from build123d import *

# Parameters (mm, degrees)
SK_BACK_PLATE_W         = 90
SK_BACK_PLATE_H         = 70
SK_BACK_PLATE_R         = 2.25
SK_BACK_PLATE_R_2       = 6
BACK_PLATE_DEPTH        = 8
SK_ROLL_PILOT_RECESS_R  = 22.15
ROLL_PILOT_RECESS_DEPTH = 2.2
SK_MEDIAL_PLATE_R       = 2.75
SK_MEDIAL_PLATE_R_2     = 13
MEDIAL_PLATE_DEPTH      = 8


with BuildPart() as part:
    # SK_Back_Plate → Back_Plate (new body)
    with BuildSketch(Plane(origin=(-76, 0, 0), x_dir=(0, 0, -1), z_dir=(1, 0, 0))):
        with Locations((0, -1)):
            Rectangle(SK_BACK_PLATE_W, SK_BACK_PLATE_H)
        with Locations((25.86862691, 10.715136106)):
            Circle(SK_BACK_PLATE_R, mode=Mode.SUBTRACT)
        with Locations((10.715136106, 25.86862691)):
            Circle(SK_BACK_PLATE_R, mode=Mode.SUBTRACT)
        with Locations((-10.715136106, 25.86862691)):
            Circle(SK_BACK_PLATE_R, mode=Mode.SUBTRACT)
        with Locations((-25.86862691, 10.715136106)):
            Circle(SK_BACK_PLATE_R, mode=Mode.SUBTRACT)
        with Locations((-25.86862691, -10.715136106)):
            Circle(SK_BACK_PLATE_R, mode=Mode.SUBTRACT)
        with Locations((-10.715136106, -25.86862691)):
            Circle(SK_BACK_PLATE_R, mode=Mode.SUBTRACT)
        with Locations((10.715136106, -25.86862691)):
            Circle(SK_BACK_PLATE_R, mode=Mode.SUBTRACT)
        with Locations((25.86862691, -10.715136106)):
            Circle(SK_BACK_PLATE_R, mode=Mode.SUBTRACT)
        Circle(SK_BACK_PLATE_R_2, mode=Mode.SUBTRACT)
    extrude(amount=BACK_PLATE_DEPTH)

    # SK_Roll_Pilot_Recess → Roll_Pilot_Recess (cut)
    with BuildSketch(Plane(origin=(-76, 0, 0), x_dir=(0, 0, -1), z_dir=(1, 0, 0))):
        Circle(SK_ROLL_PILOT_RECESS_R)
    extrude(amount=ROLL_PILOT_RECESS_DEPTH, mode=Mode.SUBTRACT)

    # SK_Medial_Plate → Medial_Plate (add)
    with BuildSketch(Plane(origin=(0, -28, 0), x_dir=(1, 0, 0), z_dir=(0, 1, 0))):
        Polygon((-68, 56), (30, 56), (56, 30), (56, -30), (30, -56), (-68, -56), align=None)
        with Locations(Location((46.193976626, 19.134171618, 0), (0, 0, 270))):
            Circle(SK_MEDIAL_PLATE_R, mode=Mode.SUBTRACT)
        with Locations(Location((19.134171618, 46.193976626, 0), (0, 0, 270))):
            Circle(SK_MEDIAL_PLATE_R, mode=Mode.SUBTRACT)
        with Locations(Location((-19.134171618, 46.193976626, 0), (0, 0, 270))):
            Circle(SK_MEDIAL_PLATE_R, mode=Mode.SUBTRACT)
        with Locations(Location((-46.193976626, 19.134171618, 0), (0, 0, 270))):
            Circle(SK_MEDIAL_PLATE_R, mode=Mode.SUBTRACT)
        with Locations(Location((-46.193976626, -19.134171618, 0), (0, 0, 270))):
            Circle(SK_MEDIAL_PLATE_R, mode=Mode.SUBTRACT)
        with Locations(Location((-19.134171618, -46.193976626, 0), (0, 0, 270))):
            Circle(SK_MEDIAL_PLATE_R, mode=Mode.SUBTRACT)
        with Locations(Location((19.134171618, -46.193976626, 0), (0, 0, 270))):
            Circle(SK_MEDIAL_PLATE_R, mode=Mode.SUBTRACT)
        with Locations(Location((46.193976626, -19.134171618, 0), (0, 0, 270))):
            Circle(SK_MEDIAL_PLATE_R, mode=Mode.SUBTRACT)
        with Locations(Location((0, 0, 0), (0, 0, 270))):
            Circle(SK_MEDIAL_PLATE_R_2, mode=Mode.SUBTRACT)
    extrude(amount=MEDIAL_PLATE_DEPTH)


solid = part.part
Could you check a few things on this model? Use its own coordinates, in mm. A direction names the side the tool comes from. Round coordinates to 2 decimals unless told otherwise and drop trailing zeros. Order: outer loops, then holes, each group sorted by start corner. A loop starts at its lowest first (then second) coordinate and runs counter-clockwise, first axis right, second up.
(1) Imagine slicing it at D-D (z = -33). Write out the boundary of the cut face in (x, y).
Response values:
outline: (-76, -36) - (-68, -36) - (-68, -28) - (53, -28) - (53, -20) - (-68, -20) - (-68, 34) - (-76, 34) - close
(2) Imagine slicing it at A-A (y = 0). Write out the boundary of the cut face in (x, z), plus the area to 3 significant figures.
Response values:
outline: (-76, -45) - (-68, -45) - (-68, -6) - (-73.8, -6) - (-73.8, -22.15) - (-76, -22.15) - close; (-76, 22.15) - (-73.8, 22.15) - (-73.8, 6) - (-68, 6) - (-68, 45) - (-76, 45) - close
area: 553 mm2
(3) Imagine slicing it at B-B (z = 0). Write out the boundary of the cut face in (x, y).
Response values:
outline: (-76, -36) - (-68, -36) - (-68, -28) - (-13, -28) - (-13, -20) - (-68, -20) - (-68, -6) - (-73.8, -6) - (-73.8, -22.15) - (-76, -22.15) - close; (-76, 22.15) - (-73.8, 22.15) - (-73.8, 6) - (-68, 6) - (-68, 34) - (-76, 34) - close; (13, -28) - (56, -28) - (56, -20) - (13, -20) - close
(4) I'm going to push flat-ended pins straight in: pin 1 (5 mm diameter, centred on x = -46.19, z = 19.13, fed in from -Y); pin 2 (2.5 mm diameter, centred on y = -25.87, z = -10.72, fed in from -X); pin 3 (1 mm diameter, centred on y = -1, z = -19.5, fed in from -X); pin 4 (7 mm diameter, centred on x = -19.13, z = -46.19, fed in from +Y). Where does each tip first touch, or does it pass through?
Response values:
pin 1: passes through
pin 2: stops at x = -68
pin 3: stops at x = -73.8
pin 4: stops at y = -20
(5) Which directions (+Z, -Z, +X, -X, +Y, -Y) give clear straight access to the entire face, cutting with the end or side of a thin tool? Please do faces 1 (the flat face through (-19, -20, -1)), 2 (the cylindrical face through (-72.06, -23.64, -10.42)), 3 (the flat face through (-68, -32, 1)).
Response values:
face 1: +Z, -Z, +X, +Y
face 2: -X
face 3: +Z, -Z, +X, -Y
(6) Imagine slicing it at C-C (x = 0). Write out the boundary of the cut face in (y, z).
Response values:
outline: (-28, -56) - (-20, -56) - (-20, -13) - (-28, -13) - close; (-28, 13) - (-20, 13) - (-20, 56) - (-28, 56) - close
(7) Please list where these lines run through material, in increasing order: line 1 along Y through (x, z) = (-67.5, -21); line 2 along X through (y, z) = (-29, 20); line 3 along Z through (x, y) = (8.5, -24).
Response values:
line 1: y = -28 to -20
line 2: x = -76 to -68
line 3: z = -56 to -9.84, 9.84 to 56
(8) If we mould it in two halves opening along Z, with no side actions, what happens to faces 4 (the cylindrical face through (-48.88, -24.06, -19.73)), 5 (the flat face through (56, -24, 0)), 6 (the flat face through (-72, -1, -45))? For each: released by +Z, released by -Z, zero draft, split by the parting line, or undercut.
Response values:
face 4: undercut
face 5: zero draft
face 6: released by -Z
